```python
from build123d import *

# Parameters (mm, degrees)
ESBO_O1_R                = 13
ESBO_O1_R_2              = 4.765
RESSALTO_EXTRUS_O1_DEPTH = 8
ESBO_O2_R                = 11
ESBO_O2_R_2              = 7
CORTE_EXTRUS_O1_DEPTH    = 1
CORTE_EXTRUS_O2_START    = -1
ESBO_O3_R                = 11
ESBO_O3_R_2              = 7
CORTE_EXTRUS_O2_DEPTH    = 1
FILETE1_R                = 1


with BuildPart() as part:
    # Esboço1 → Ressalto-extrusão1 (new body)
    with BuildSketch(Plane.XY):
        Circle(ESBO_O1_R)
        Circle(ESBO_O1_R_2, mode=Mode.SUBTRACT)
    extrude(amount=RESSALTO_EXTRUS_O1_DEPTH)

    # Esboço2 → Corte-extrusão1 (cut)
    with BuildSketch(Plane.XY.offset(8)):
        Circle(ESBO_O2_R)
        Circle(ESBO_O2_R_2, mode=Mode.SUBTRACT)
    extrude(amount=-CORTE_EXTRUS_O1_DEPTH, mode=Mode.SUBTRACT)

    # Esboço3 → Corte-extrusão2 (cut)
    with BuildSketch(Plane(origin=(0, 0, 0), x_dir=(-1, 0, 0), z_dir=(0, 0, -1)).offset(CORTE_EXTRUS_O2_START)):
        with Locations(Location((0, 0, 0), (0, 0, 180))):
            Circle(ESBO_O3_R)
        with Locations(Location((0, 0, 0), (0, 0, 180))):
            Circle(ESBO_O3_R_2, mode=Mode.SUBTRACT)
    extrude(amount=CORTE_EXTRUS_O2_DEPTH, mode=Mode.SUBTRACT)

    # Filete1
    filete1_edges = [part.edges().sort_by_distance(p)[0] for p in [
        (-13, 0, 0),
        (-13, 0, 8),
    ]]
    fillet(filete1_edges, radius=FILETE1_R)


solid = part.part
```
Build history of the part. All positions in model axes, mm. A direction names the side the tool comes from. Give positions to 0.01 mm unless a question says otherwise; leave off trailing zeros. Order: outer loops, then holes, each group sorted by start corner. A loop starts at its lowest first (then second) coordinate and runs counter-clockwise, first axis right, second up. Notation, with made-up numbers: M -11.75,5.5 L 35.25,5.5 A13 cw 35.25,11.5 Z; hole C -6.5,38 d3. An arc over 180 degrees is marked long. Return JSON: item names as keys, results as strings.
Q1. Wall check: probe 1 along Y at (x, z) = (0, 0.55) (3 decimals); probe 2 along Y at (x, z) = (0, 5) (3 decimals); probe 3 along Y at (x, z) = (0, 7.3) (3 decimals). Give the ranges that are in metal, low to high. Write a range as from..to.
Answer list:
{"probe 1": "y = -12.893..-11, -7..-4.765, 4.765..7, 11..12.893", "probe 2": "y = -13..-4.765, 4.765..13", "probe 3": "y = -12.954..-11, -7..-4.765, 4.765..7, 11..12.954"}
Q2. 3-axis set-ups, long thin cutter, end or side, ignore diameter. For faces 1 (the face through (1, -5, 0)), 2 (the face through (-2.38, 10.74, 0.51)), 3 (the face through (7.2, 0.2, 7)): which of +Z, -Z, +X, -X, +Y, -Y reach the whole face in a straight line?
Answer list:
{"face 1": "-Z, +X, -X, +Y, -Y", "face 2": "-Z", "face 3": "+Z"}
Q3. Band-saw the part on C-C (z = 4). Give the cut face in (x, y) (3 decimals), then the cut area to 3 significant figures.
Answer list:
{"outline": "C 0,0 d26; hole C 0,0 d9.53", "area": "460 mm^2"}
Q4. Two-plate mould, pull along Y, no slides. Class faces 4 (the face through (5, -10, 8)), 5 (the face through (-10.316, -7.91, 3.958)), 6 (the face through (6.466, -2.681, 7.507)): pulls with the +Y half, pulls with the -Y half, needs draft (parallel to the pull), parting line crosses it, or undercut.
Answer list:
{"face 4": "needs draft", "face 5": "parting line crosses it", "face 6": "undercut"}
Q5. Band-saw the part on A-A (y = 0). Give the cut face in (x, z) (3 decimals).
Answer list:
{"outline": "M -13,1 A1 ccw -12,0 L -11,0 L -11,1 L -7,1 L -7,0 L -4.765,0 L -4.765,8 L -7,8 L -7,7 L -11,7 L -11,8 L -12,8 A1 ccw -13,7 Z; M 4.765,0 L 7,0 L 7,1 L 11,1 L 11,0 L 12,0 A1 ccw 13,1 L 13,7 A1 ccw 12,8 L 11,8 L 11,7 L 7,7 L 7,8 L 4.765,8 Z"}
Q6. Flat gauge pins, fed straight in: pin 1 (1.5 mm diameter, centred on y = 3, z = 2, fed in from -X); pin 2 (4 mm diameter, centred on x = -9.5, z = 4.5, fed in from +Y). Where does each tip first touch, or does it go through?
Answer list:
{"pin 1": "stops at x = -12.8", "pin 2": "stops at y = 10.62"}
